Read the model definition and answer for the solid it produces. Units are mm, in the model's axes. A direction names the side the tool comes from. Round coordinates to 2 decimals unless told otherwise and drop trailing zeros. Write each loop counter-clockwise with the first axis right and the second up, starting at its lowest first coordinate (ties: lowest second). Pieces come first, ordered by that corner, then holes. Notation, with made-up numbers: (74.5, 9) - (122.5, 9) arc R20 cw to (122.5, 39) - close; hole circle Ø3 at (77, -4). An arc over 180 degrees is marked (long way). One line per item, written item: value. Start each with the question number.
(1) Flat-ended cylindrical pins translate along their axes: pin 1 Ø1.8 at (y, z) = (-18.295, 0) entering from -X; pin 2 Ø0.5 at (x, y) = (0, -54.5) entering from -Z. Find the tip coordinate at first contact, or state that the pin passes through.
(2) Find the intervals of material crossed by L1, parallel to Z at x = -0.7, y = -18.5; L2, parallel to Z at x = 0.75, y = -58.5; L3, parallel to Y at x = -0.55, z = -6 (3 decimals), in increasing order.
(3) A cutting plane is placed at A-A, the plane x = 0.1. Determine the outline of the cut face in (y, z) (3 decimals).
(4) For faces 1 (the face through (0, -100.745, -5)), 2 (the face through (0.011, -51.128, -0.505)), determine the directions among +Z, -Z, +X, -X, +Y, -Y from which every point of the face is accessible in a straight line to the end or side of a thin tool.
(5) The mould has two halves that part along Y. Classify faces 3 (the face through (0.01, -64.1, -14.53)), 4 (the face through (0, -82, -15)), 5 (the face through (-0.011, -11.365, -14.399)): +Y half, -Y half, draft (parallel to the pull), parting line (faces both ways), or undercut.
from build123d import *

# Parameters (mm, degrees)
SKETCH_1_R      = 1.1303
EXTRUDE_1_DEPTH = 1.588
FILLET_1_R      = 2
FILLET_2_R      = 2
FILLET_3_R      = 2
FILLET_4_R      = 2


with BuildPart() as part:
    # 草图1 → 凸台-拉伸1 (new body)
    with BuildSketch(Plane(origin=(-0.79375, 0, 0), x_dir=(0, -1, 0), z_dir=(-1, 0, 0))):
        with BuildLine():
            Line((38.795, 5), (12.795, 5))
            ThreePointArc((12.795, 5), (11.380786438, 4.414213562), (10.795, 3))
            Line((10.795, 3), (10.795, -13))
            ThreePointArc((10.795, -13), (11.380786438, -14.414213562), (12.795, -15))
            Line((12.795, -15), (47.795, -15))
            Line((47.795, -15), (50.77, -0.039144756))
            Line((50.77, -0.039144756), (55.77, -0.039144756))
            Line((55.77, -0.039144756), (60.77, -0.039144756))
            Line((60.77, -0.039144756), (63.745, -15))
            Line((63.745, -15), (98.745, -15))
            ThreePointArc((98.745, -15), (100.159213562, -14.414213562), (100.745, -13))
            Line((100.745, -13), (100.745, 3))
            ThreePointArc((100.745, 3), (100.159213562, 4.414213562), (98.745, 5))
            Line((98.745, 5), (72.745, 5))
            Line((72.745, 5), (38.795, 5))
        make_face()
        with Locations((18.295, 0)):
            Circle(SKETCH_1_R, mode=Mode.SUBTRACT)
        with Locations((13.295, 0)):
            Circle(SKETCH_1_R, mode=Mode.SUBTRACT)
        with Locations((98.245, 0)):
            Circle(SKETCH_1_R, mode=Mode.SUBTRACT)
        with Locations((93.245, 0)):
            Circle(SKETCH_1_R, mode=Mode.SUBTRACT)
    extrude(amount=-EXTRUDE_1_DEPTH)

    # 圆角1
    fillet_1_edges = [part.edges().sort_by_distance(p)[0] for p in [
        (0.00025, -50.77, -0.039144756),
    ]]
    fillet(fillet_1_edges, radius=FILLET_1_R)

    # 圆角2
    fillet_2_edges = [part.edges().sort_by_distance(p)[0] for p in [
        (0.00025, -47.795, -15),
    ]]
    fillet(fillet_2_edges, radius=FILLET_2_R)

    # 圆角3
    fillet_3_edges = [part.edges().sort_by_distance(p)[0] for p in [
        (0.00025, -60.77, -0.039144756),
    ]]
    fillet(fillet_3_edges, radius=FILLET_3_R)

    # 圆角4
    fillet_4_edges = [part.edges().sort_by_distance(p)[0] for p in [
        (0.00025, -63.745, -15),
    ]]
    fillet(fillet_4_edges, radius=FILLET_4_R)


solid = part.part
Here are the results:
1. pin 1: through
1. pin 2: z = -0.04
2. L1: -15 to -1.11, 1.11 to 5
2. L2: -0.04 to 5
2. L3: -100.745 to -61.955, -49.585 to -10.795
3. outline: (-100.745, -13) arc R2 ccw to (-98.745, -15) - (-65.386, -15) arc R2 ccw to (-63.425, -13.39) - (-61.09, -1.649) arc R2 cw to (-59.129, -0.039) - (-52.411, -0.039) arc R2 cw to (-50.45, -1.649) - (-48.115, -13.39) arc R2 ccw to (-46.154, -15) - (-12.795, -15) arc R2 ccw to (-10.795, -13) - (-10.795, 3) arc R2 ccw to (-12.795, 5) - (-98.745, 5) arc R2 ccw to (-100.745, 3) - close; hole circle Ø2.261 at (-98.245, 0); hole circle Ø2.261 at (-93.245, 0); hole circle Ø2.261 at (-18.295, 0); hole circle Ø2.261 at (-13.295, 0)
4. face 1: +Z, -Z, +X, -X, -Y
4. face 2: -Z, +X, -X
5. face 3: undercut
5. face 4: draft
5. face 5: +Y half
